Autodesk Inventor part; units mm, degrees
ref_plane "YZ Plane" through (0, 0, 0) normal (1, 0, 0) x (0, 1, 0)
ref_plane "XZ Plane" through (0, 0, 0) normal (0, 1, 0) x (-1, 0, 0)
ref_plane "XY Plane" through (0, 0, 0) normal (0, 0, 1) x (1, 0, 0)
sketch "Sketch1" plane through (0, 0, 0) normal (0, 1, 0) x (-1, 0, 0)
  line L0 (0, 0) -> (-3.8165, 0)
  line L1 (-3.8165, 0) -> (-3.1049, -0.7116)
  line L2 (-3.1049, -0.7116) -> (-3.1049, -2.701)
  arc A0 (-3.1049, -2.701) -> (-1.6284, -4.75) centre (-0.9449, -2.701) ccw
  line L3 (-0.9449, -5.6986) -> (-0.9449, -8.55)
  line L4 (-1.9449, -9.55) -> (-4.5949, -9.55)
  line L5 (-5.5949, -8.55) -> (-5.5949, -5.75)
  line L6 (-6.5949, -4.75) -> (-7.0833, -4.75)
  line L7 (-7.0833, -4.75) -> (-7.7949, -4.0384)
  line L8 (-7.7949, -4.0384) -> (-7.7949, -0.7116)
  line L9 (-7.7949, -0.7116) -> (-7.0833, 0)
  line L10 (-7.0833, 0) -> (-3.8165, 0)
  circle A1 centre (-5.4499, -2.1243) radius 1.45
  circle A2 centre (-3.2499, -7.1243) radius 1.45
  arc A3 (-0.9449, -5.6986) -> (-1.6284, -4.75) centre (-1.9449, -5.6986) ccw
  arc A4 (-5.5949, -5.75) -> (-6.5949, -4.75) centre (-6.5949, -5.75) ccw
  arc A5 (-1.9449, -9.55) -> (-0.9449, -8.55) centre (-1.9449, -8.55) ccw
  arc A6 (-5.5949, -8.55) -> (-4.5949, -9.55) centre (-4.5949, -8.55) ccw
  point P0 (-0.9449, -4.861)
  point P1 (-5.5949, -7.15)
  point P2 (-5.4499, 0)
  point P3 (-6.8391, -4.75)
  point P4 (-0.9449, -7.1243)
  dimension "d0" = 5
  dimension "d1" = 2.2
  dimension "d2" = 2.9
  dimension "d3" = 4.75
  dimension "d4" = 4.65
  dimension "d6" = 4.69
  dimension "d8" = 6.85
  dimension "d9" = 9.55
  dimension "d10" = 135
  dimension "d11" = 135
  dimension "d12" = 135
  dimension "d13" = 1
  dimension "d14" = 1
extrude "Extrusion1" add sketch "Sketch1" along normal blind 1.8 contours L1 L2 A0 A3 L3 A5 L4 A6 L5 A4 L6 L7 L8 L9 L10 | A1 | A2
extrude "Extrusion2" add sketch "Sketch1" against normal blind 1.25 contours A1 | A2
chamfer "Chamfer1" distance 0.1 angle 45 2 edges at (6.8999, -1.25, -2.1243) (4.6999, -1.25, -7.1243)
sketch "Sketch2" plane through (3.8165, 0, 0) normal (0, 0, 1) x (1, 0, 0)
  line L0 (1.7784, 1.8) -> (2.7784, 1.8)
  line L1 (2.4734, -0.05) -> (0.7934, -0.05)
  line L2 (0.7784, 0) -> (0.7784, 1.8)
  line L3 (3.2668, 0) -> (3.2668, 1.8)
  line L4 (0, 0) -> (0, 1.8)
  line L5 (0, 1.8) -> (3.2668, 1.8)
  line L6 (2.4734, -0.05) -> (2.4734, 1.7)
  line L7 (0.7934, -0.05) -> (0.7934, 1.7)
  line L8 (0.8934, 1.7) -> (0.8934, 0.05)
  line L9 (0.8934, 0.05) -> (2.3734, 0.05)
  line L10 (2.3734, 0.05) -> (2.3734, 1.7)
  line L11 (2.4734, 1.7) -> (2.3734, 1.7)
  line L12 (0.8934, 1.7) -> (0.7934, 1.7)
  point P0 (-3.8165, 0)
  dimension "d24" = 1.68
  dimension "d26" = 1.85
  dimension "d27" = 0.1
  dimension "d28" = 0.7934
  dimension "d29" = 0.7934
  dimension "d30" = 0.1
  dimension "d31" = 0.1
extrude "Extrusion3" add sketch "Sketch2" along normal blind 1.8
sketch "Sketch3" plane through (4.6099, 0, 0) normal (-1, 0, 0) x (0, 0, 1)
  line L0 (0, -0.05) -> (1.8, -0.05)
  line L1 (0.16, -0.05) -> (0.16, 0.54)
  line L2 (0, 0) -> (0, 1.7)
  arc A0 (0.16, 0.54) -> (0, 0.7) centre (0, 0.54) ccw
  line L3 (0, 0) -> (0, 1.8)
  line L4 (0, 0) -> (0, 1.7)
  line L5 (0, 0) -> (0, -0.05)
  line L6 (0, -0.05) -> (1.8, -0.05)
  line L7 (1.8, 1.7) -> (1.8, -0.05)
  line L8 (0, 1.7) -> (1.8, 1.7)
  point P0 (0, 0)
  dimension "d34" = 0.16
  dimension "d54" = 0.75
extrude "Extrusion4" cut sketch "Sketch3" against normal through all contours L5 L2 A0 L1 L0
sketch "Sketch4" plane through (4.5949, 0, -9.55) normal (0, 0, -1) x (-1, 0, 0)
  line L0 (2.165, -0.05) -> (0.485, -0.05)
  line L1 (2.165, -0.05) -> (2.165, 1.7)
  line L2 (0.485, -0.05) -> (0.485, 1.7)
  line L3 (0.585, 1.7) -> (0.585, 0.05)
  line L4 (0.585, 0.05) -> (2.065, 0.05)
  line L5 (2.065, 0.05) -> (2.065, 1.7)
  line L6 (2.165, 1.7) -> (2.065, 1.7)
  line L7 (0.585, 1.7) -> (0.485, 1.7)
  line L8 (2.65, 0) -> (2.65, 1.8)
  line L9 (0, 1.8) -> (2.65, 1.8)
  line L10 (0, 0) -> (0, 1.8)
  point P0 (4.5949, 0)
  dimension "d37" = 1.68
  dimension "d42" = 0.1
  dimension "d43" = 0.1
  dimension "d44" = 0.485
  dimension "d45" = 0.485
  dimension "d46" = 1.85
  dimension "d47" = 0.1
extrude "Extrusion5" add sketch "Sketch4" along normal blind 1.8
sketch "Sketch5" plane through (2.4299, 0, -9.55) normal (-1, 0, 0) x (0, 0, 1)
  line L0 (0, -0.05) -> (0, 0)
  line L1 (0, 1.7) -> (0, 0)
  line L2 (0, 1.7) -> (-1.8, 1.7)
  line L3 (-1.8, -0.05) -> (-1.8, 1.7)
  line L4 (0, -0.05) -> (-1.8, -0.05)
  line L5 (-0.16, -0.05) -> (-0.16, 0.54)
  arc A0 (0, 0.7) -> (-0.16, 0.54) centre (0, 0.54) ccw
  point P0 (9.55, 0)
  point P1 (-1.867, -0.613)
  point P2 (-1.867, -0.6608)
  point P3 (0, -0.025)
  dimension "d51" = 0.16
  dimension "d55" = 0.75
extrude "Extrusion6" cut sketch "Sketch5" against normal through all contours L4 L5 A0 L1 L0
sketch "Sketch6" plane through (5.4499, -1.25, -2.1243) normal (0, -1, 0) x (1, 0, 0)
  line L0 (0.1, 0.6) -> (-0.1, 0.6)
  line L1 (-0.1, 0.6) -> (-0.1, -0.6)
  line L2 (-0.1, -0.6) -> (0.1, -0.6)
  line L3 (0.1, -0.6) -> (0.1, 0.6)
  line L4 (-2.1, -4.4) -> (-2.3, -4.4)
  line L5 (-2.3, -4.4) -> (-2.3, -5.6)
  line L6 (-2.3, -5.6) -> (-2.1, -5.6)
  line L7 (-2.1, -5.6) -> (-2.1, -4.4)
  circle A0 centre (0, 0) radius 1.35
  circle A1 centre (-2.2, -5) radius 1.35
  point P0 (-5.4499, 2.1243)
  point P1 (0.1, 0)
  point P2 (0, 0.6)
  point P3 (-2.1, -5)
  point P4 (-2.2, -4.4)
  dimension "d56" = 1.2
  dimension "d57" = 0.2
  dimension "d58" = 1.2
  dimension "d59" = 0.2
extrude "Extrusion7" cut sketch "Sketch6" against normal through all contours L3 L2 L1 L0 | L7 L6 L5 L4
chamfer "Chamfer2" distance 0.2 angle 45 8 edges at (5.5499, -1.25, -2.1243) (5.4499, -1.25, -1.5243) (5.3499, -1.25, -2.1243) (5.4499, -1.25, -2.7243) (3.3499, -1.25, -7.1243) (3.2499, -1.25, -6.5243) (3.1499, -1.25, -7.1243) (3.2499, -1.25, -7.7243)
fillet "Fillet1" radius 0.4 8 edges at (4.6099, -0.05, 0.98) (6.2899, -0.05, 0.98) (6.1899, 0.05, 0.98) (4.7099, 0.05, 0.98) (2.4299, -0.05, -10.53) (4.1099, -0.05, -10.53) (4.0099, 0.05, -10.53) (2.5299, 0.05, -10.53)
equation "\"d11\" = d10"
equation "\"d29\" = d28"
properties part number "Kailh Choc Hotswap Socket Negative"
Geometry: final body of the model. Coordinates: model frame, mm. A direction names the side the tool comes from. Coordinates: 2 decimals unless noted, no trailing zeros. Order: outer loops, then holes, each group sorted by start corner. A loop starts at its lowest first (then second) coordinate and runs counter-clockwise, first axis right, second up. Notation, with made-up numbers: (15, -22.5) -> (47, -22.5) arc R16 ccw to (47, -13.5) -> close; hole circle Ø10 at (20.5, 7). An arc over 180 degrees is marked (long way). Answer in a Markdown table with one row per item.
Item 1: Contact query for flat-ended pins moving along their axis: P1, Ø0.5, axis at x = 3, z = -11, coming from the +Y side; P2, Ø1, axis at y = 1, z = -11, coming from the -X side; P3, Ø0.6, axis at y = 1, z = 1, coming from the +X side. Output: stop coordinate, or through.
Return value:
| item | result |
|---|---|
| P1 | stops at y = 0.09 |
| P2 | stops at x = 2.43 |
| P3 | stops at x = 6.29 |
Item 2: Section D-D on z = -5.5. Output: boundary loops of the cut face in (x, y).
Return value:
| item | result |
|---|---|
| outline | (0.96, 0) -> (5.63, 0) -> (5.63, 1.8) -> (0.96, 1.8) -> close |
Item 3: Ray query, L1, parallel to Y at x = 3.5, z = -4.5; L2, parallel to X at y = -0.5, z = -7; L3, parallel to Z at x = 4.5, y = 1.4. Return the intervals inside material, ascending.
Return value:
| item | result |
|---|---|
| L1 | y = 0 to 1.8 |
| L2 | x = 1.81 to 3.15, 3.35 to 4.69 |
| L3 | z = -9.55 to 0 |
Item 4: Section C-C on x = 1.5. Output: boundary loops of the cut face in (y, z), plus the area to 3 significant figures.
Return value:
| item | result |
|---|---|
| outline | (0, -9.45) -> (1.8, -9.45) -> (1.8, -4.8) -> (0, -4.8) -> close |
| area | 8.36 mm² |
Item 5: Access query for faces 1 (the flat face through (7.795, 1, -2)), 2 (the cylindrical face through (1.91, -0.57, -7.68)), 3 (the flat face through (5.595, 1, -7)), 4 (the flat face through (3.105, 1, -2)), 5 (the flat face through (5.55, 0, -2)). Directions: +Z, -Z, +X, -X, +Y, -Y. A direction counts if a zero-diameter tool reaches every point of the face in a straight line with its end or side. Return the directions, or none.
Return value:
| item | result |
|---|---|
| face 1 | +Z, -Z, +X, +Y, -Y |
| face 2 | -Y |
| face 3 | -Z, +X, +Y, -Y |
| face 4 | +Z, -X, +Y, -Y |
| face 5 | +Y, -Y |
Item 6: Section A-A on y = -0.7. Output: boundary loops of the cut face in (x, z), plus the area to 3 significant figures.
Return value:
| item | result |
|---|---|
| outline | circle Ø2.9 at (3.25, -7.12); circle Ø2.9 at (5.45, -2.12); hole (3.15, -7.72) -> (3.35, -7.72) -> (3.35, -6.52) -> (3.15, -6.52) -> close; hole (5.35, -2.72) -> (5.55, -2.72) -> (5.55, -1.52) -> (5.35, -1.52) -> close |
| area | 12.7 mm² |
Item 7: Section B-B on z = -10.5. Output: boundary loops of the cut face in (x, y).
Return value:
| item | result |
|---|---|
| outline | (2.43, 0.35) arc R0.4 ccw to (2.83, -0.05) -> (3.71, -0.05) arc R0.4 ccw to (4.11, 0.35) -> (4.11, 1.7) -> (4.01, 1.7) -> (4.01, 0.45) arc R0.4 cw to (3.61, 0.05) -> (2.93, 0.05) arc R0.4 cw to (2.53, 0.45) -> (2.53, 1.7) -> (2.43, 1.7) -> close |
